For this review, take the finished solid that the model builds, in its own axes (mm). A direction names the side the tool comes from. Give positions to 0.01 mm unless a question says otherwise; leave off trailing zeros. Write each loop counter-clockwise with the first axis right and the second up, starting at its lowest first coordinate (ties: lowest second). Pieces come first, ordered by that corner, then holes.
1) For P1, Ø3, axis at x = 5, z = 11, coming from the +Y side; P2, Ø12, axis at x = 37, z = 12.5, coming from the +Y side; P3, Ø10, axis at y = -9.5, z = 5.5, coming from the -X side, all flat-tipped, find the tip position at first contact; note any pin that passes through.
2) Draft analysis for pull direction X (two halves, no side actions). For faces 3 (the face through (-19.79, -45.94, 7.4)), 4 (the face through (27.561, -14.428, 7.395)), 5 (the face through (-25, -17, 15)), state which applies: pulls with the +X half, pulls with the -X half, needs draft (parallel to the pull), parting line crosses it, or undercut.
3) We need section A-A on x = 25.5. Give the boundary of the cut face in (y, z) (3 decimals), and give its area (3 significant figures).
4) Wall thickness on line 1 along X through (y, z) = (21, 13.75); line 2 along X through (y, z) = (20, 7); line 3 along Y through (x, z) = (18.5, 6.25): over which ranges is each line inside the solid? List them lowest first.
5) We need section D-D on y = -12. Give the boundary of the cut face in (x, z), and give its area (3 significant figures).
6) Machinability: for faces 1 (the face through (30.387, 6.664, 7.395)), 2 (the face through (34.31, 36.4, 7.4)), which of the approach directions +Z, -Z, +X, -X, +Y, -Y give a long, thin tool a straight path to every point of the face, cutting with its end or side? Answer none if there is none.
7) We need section C-C on y = 0. Give the boundary of the cut face in (x, z).
8) We need section B-B on z = 1.25. Give the number of separate pieces and of enclosed holes in the cut face, and give its area (3 significant figures).
from build123d import *

# Parameters (mm, degrees)
SKETCH_R           = 50
PAD_DEPTH          = 5
PAD001_DEPTH       = 15
POLARPATTERN_COUNT = 9


with BuildPart() as part:
    # Sketch → Pad (new body)
    with BuildSketch(Plane.XY):
        Circle(SKETCH_R)
    extrude(amount=-PAD_DEPTH)

    # Sketch001 → Pad001 (join)
    with BuildSketch(Plane.XY):
        with BuildLine():
            ThreePointArc((43.30127, -25), (29.522789, -9.6465), (10.718625, -1.162401))
            ThreePointArc((9.015743, -5.912401), (10.148987, -3.638428), (10.718625, -1.162401))
            ThreePointArc((40.186285, -29.75), (27.336197, -14.254618), (9.015743, -5.912401))
            ThreePointArc((40.186285, -29.75), (41.829839, -27.431438), (43.30127, -25))
        make_face()
    pad001 = extrude(amount=PAD001_DEPTH)

    # PolarPattern: Pad001 ×9 about axis
    polarpattern_axis = Axis((0, 0, 0), (0, 0, 1))
    for i in range(1, POLARPATTERN_COUNT):
        add(pad001.rotate(polarpattern_axis, i * 360 / POLARPATTERN_COUNT))


solid = part.part
Results list:
1. P1: stops at y = 49.9
1. P2: stops at y = 38.3
1. P3: stops at x = -21.74
2. face 3: pulls with the -X half
2. face 4: undercut
2. face 5: needs draft
3. outline: (-43.009, -5) - (43.009, -5) - (43.009, 0) - (35.322, 0) - (35.322, 15) - (29.546, 15) - (29.546, 0) - (11.255, 0) - (11.255, 15) - (6.205, 15) - (6.205, 0) - (-6.991, 0) - (-6.991, 15) - (-12.922, 15) - (-12.922, 0) - (-43.009, 0) - close
3. area: 681 mm2
4. line 1: x = -25.62 to -19.64, -6.54 to -1.52, 9 to 15.42
4. line 2: x = -24.99 to -18.91, -6.45 to -1.42, 8.29 to 14.57
4. line 3: y = -8.98 to -3.55, 4.58 to 9.8, 24.18 to 30.75
5. outline: (-48.54, -5) - (48.54, -5) - (48.54, 0) - (32.5, 0) - (32.5, 15) - (24.1, 15) - (24.1, 0) - (10.38, 0) - (10.38, 15) - (4.37, 15) - (4.37, 0) - (0.65, 0) - (0.65, 15) - (-4.36, 15) - (-4.36, 0) - (-9.67, 0) - (-9.67, 15) - (-17.69, 15) - (-17.69, 0) - (-48.54, 0) - close
5. area: 897 mm2
6. face 1: +Z
6. face 2: +Z, -Z, +X, +Y
7. outline: (-50, -5) - (50, -5) - (50, 0) - (-10.78, 0) - (-10.78, 15) - (-34.2, 15) - (-34.2, 0) - (-50, 0) - close
8. separate pieces: 9
8. enclosed holes: 0
8. area: 1,840 mm2
